Can you work these out from the model? Positions are in its coordinate system, mm. A direction names the side the tool comes from. Give positions to 0.01 mm unless a question says otherwise; leave off trailing zeros. Order: outer loops, then holes, each group sorted by start corner. A loop starts at its lowest first (then second) coordinate and runs counter-clockwise, first axis right, second up. Notation, with made-up numbers: (83.25, -5.5) - (137.25, -5.5) arc R21 cw to (137.25, 19.5) - close; hole circle Ø7 at (80.5, -16.5). An arc over 180 degrees is marked (long way). Return JSON: item names as keys, results as strings.
```python
from build123d import *

# Parameters (mm, degrees)
BOX006_W               = 85
BOX006_H               = 10
BOX006_DEPTH           = 10
ARRAY_X_COUNT          = 2
ARRAY_X_PITCH          = 100
ARRAY_Y_COUNT          = 8
ARRAY_Y_PITCH          = 16
BOX004_W               = 220
BOX004_H               = 36
BOX004_DEPTH           = 10
BOX005_W               = 220
BOX005_H               = 10
BOX005_DEPTH           = 27
BOX003_W               = 198
BOX003_H               = 14.14
BOX003_DEPTH           = 14.14
BOX003_ROLL_ANGLE      = 45
CUT001_PLACEMENT_ANGLE = 180
BOX001_W               = 198
BOX001_H               = 4
BOX001_DEPTH           = 10
BOX002_W               = 205
BOX002_H               = 3
BOX002_DEPTH           = 3
BOX_W                  = 210
BOX_H                  = 153.85
BOX_DEPTH              = 2


with BuildPart() as array:
    # Box006 → Box006 (new body)
    with BuildSketch(Plane(origin=(12.5, 14, 0), x_dir=(1, 0, 0), z_dir=(0, 0, 1))):
        with Locations((42.5, 5)):
            Rectangle(BOX006_W, BOX006_H)
    extrude(amount=BOX006_DEPTH)

    # Array X: Array ×2


with BuildPart() as array_1:
    add(array.part)
    with Locations(*[(i * ARRAY_X_PITCH, 0, 0) for i in range(1, ARRAY_X_COUNT)]):
        add(array.part)

    # Array Y: Array ×8


with BuildPart() as array_2:
    add(array_1.part)
    with Locations(*[(0, i * ARRAY_Y_PITCH, 0) for i in range(1, ARRAY_Y_COUNT)]):
        add(array_1.part)


with BuildPart() as array_3:
    # Array placement: moved
    add(array_2.part.moved(Location((0, 0, -4))))


with BuildPart() as cube001:
    # Box004 → Box004 (new body)
    with BuildSketch(Plane(origin=(-6, 76, 40), x_dir=(1, 0, 0), z_dir=(0, 0, 1))):
        with Locations((110, 18)):
            Rectangle(BOX004_W, BOX004_H)
    extrude(amount=BOX004_DEPTH)


with BuildPart() as cube002:
    # Box005 → Box005 (new body)
    with BuildSketch(Plane(origin=(-7, 110, 72), x_dir=(1, 0, 0), z_dir=(0, 0, -1))):
        with Locations((110, 5)):
            Rectangle(BOX005_W, BOX005_H)
    extrude(amount=BOX005_DEPTH)


with BuildPart() as cut001:
    # Box003 → Box003 (new body)
    with BuildSketch(Plane.XY):
        with Locations((99, 7.07)):
            Rectangle(BOX003_W, BOX003_H)
    extrude(amount=BOX003_DEPTH)


with BuildPart() as cut001_1:
    # Box003 roll: moved
    add(cut001.part.rotate(Axis((0, 0, 0), (1, 0, 0)), BOX003_ROLL_ANGLE))


with BuildPart() as cut001_2:
    # Box003 placement: moved
    add(cut001_1.part.moved(Location((0, 100, 40))))

    # Cut: cut Cube002
    add(cube002.part, mode=Mode.SUBTRACT)

    # Cut001: cut Cube001
    add(cube001.part, mode=Mode.SUBTRACT)


with BuildPart() as cut001_3:
    # Cut001 placement: moved
    add(cut001_2.part.moved(Location((210, 51.85, 50))).rotate(Axis((210, 51.85, 50), (0, 1, 0)), CUT001_PLACEMENT_ANGLE))


with BuildPart() as fusion002002:
    # Box001 → Box001 (new body)
    with BuildSketch(Plane(origin=(12, 151.85, -10), x_dir=(1, 0, 0), z_dir=(0, 0, 1))):
        with Locations((99, 2)):
            Rectangle(BOX001_W, BOX001_H)
    extrude(amount=BOX001_DEPTH)

    # Fusion002002: union Cut001
    add(cut001_3.part)


with BuildPart() as fusion002002_1:
    # Fusion002002 placement: moved
    add(fusion002002.part.moved(Location((0, -4, 0))))


with BuildPart() as obj1:
    # Box002 → Box002 (new body)
    with BuildSketch(Plane(origin=(5, 3, -3), x_dir=(1, 0, 0), z_dir=(0, 0, 1))):
        with Locations((102.5, 1.5)):
            Rectangle(BOX002_W, BOX002_H)
    extrude(amount=BOX002_DEPTH)


with BuildPart() as cut002:
    # Box → Box (new body)
    with BuildSketch(Plane.XY):
        with Locations((105, 76.925)):
            Rectangle(BOX_W, BOX_H)
    extrude(amount=BOX_DEPTH)

    # Fusion: union obj1
    add(obj1.part)

    # Fusion002003: union Fusion002002
    add(fusion002002_1.part)

    # Cut002: cut Array
    add(array_3.part, mode=Mode.SUBTRACT)


solid = cut002.part
```
1. Thinking about a two-plate mould opening in Y: for faces 1 (the face through (112.386, 142.921, -5.068)), 2 (the face through (110, 151.85, -5)), 3 (the face through (210, 93.7, 0.4)), which applies, +Y half, -Y half, draft (parallel to the pull), parting line (faces both ways), or undercut?
Checks:
{"face 1": "undercut", "face 2": "+Y half", "face 3": "draft"}
2. If I drill on L1, parallel to Z at x = 104.5, y = 79; L2, parallel to Y at x = 195, z = -1; L3, parallel to X at y = 144, z = -0.5, over which ranges is the centre line in solid material (lowest first)? Write a range as [from, to].
Checks:
{"L1": "[0, 2]", "L2": "[3, 6], [138.85, 151.85]", "L3": "[12, 210]"}
3. On a 3-axis mill with a long thin cutter (end or side, diameter ignored), from which of +Z, -Z, +X, -X, +Y, -Y can I reach the whole of each face in a straight line? I mean faces 4 (the face through (104, 61, 2)), 5 (the face through (12, 147, -3)). Say none if no direction works.
Checks:
{"face 4": "+Z, +X, -X, +Y, -Y", "face 5": "-Z, -X, +Y"}
4. Suppose I cut it at C-C (y = 11). List the corners of the cut face in (x, z) for me.
Checks:
{"outline": "(0, 0) - (210, 0) - (210, 2) - (0, 2) - close"}
5. Suppose I cut it at B-B (x = 15.5). State how many separate pieces and enclosed holes the cut face has, plus the area to 3 significant figures.
Checks:
{"separate pieces": "9", "enclosed holes": "0", "area": "247 mm^2"}
6. Suppose I cut it at A-A (y = 69.5). List the corners of the cut face in (x, z) for me, plus the area to 3 significant figures.
Checks:
{"outline": "(0, 0) - (12.5, 0) - (12.5, 2) - (0, 2) - close; (97.5, 0) - (112.5, 0) - (112.5, 2) - (97.5, 2) - close; (197.5, 0) - (210, 0) - (210, 2) - (197.5, 2) - close", "area": "80.0 mm^2"}
7. For pin 1 Ø1 at (x, z) = (74.5, -6) entering from -Y, with a flat end and sliding along its axis, tell me the tip position at first contact or that it passes through.
Checks:
{"pin 1": "y = 143.35"}
8. Suppose I cut it at D-D (z = -6.25). List the corners of the cut face in (x, y) for me.
Checks:
{"outline": "(12, 144.1) - (210, 144.1) - (210, 151.85) - (12, 151.85) - close"}
